Design review of the part built by this model. Coordinates are the model's own, in mm. Round coordinates to 2 decimals unless told otherwise and drop trailing zeros. Loops run counter-clockwise (first coordinate to the right, second up) from the corner with the lowest first, then second, coordinate; pieces in that order, holes last. Notation, with made-up numbers: (79.5, 49.5) - (85.5, 49.5) arc R14 ccw to (85.5, 67.5) - close; hole circle Ø6 at (82.5, -19.5). An arc over 180 degrees is marked (long way). Use one line per item in the form item = value. Start each with the question number.
(1) For pin 1 (4 mm diameter, centred on x = 507.5, z = 30, fed in from -Y); pin 2 (3.5 mm diameter, centred on x = -250, y = 337.5, fed in from +Z), all flat-tipped, find the tip position at first contact; note any pin that passes through.
(2) Wall thickness on probe 1 along X at (y, z) = (337.5, 28.5); probe 2 along Y at (x, z) = (-250, 28); probe 3 along X at (y, z) = (-359.5, 22): over which ranges is each line inside the solid? List them lowest first. Write a range as [from, to].
(3) We need section C-C, the plane x = -824.5. Write out the cut boundary in (y, z), then the cut area to 3 significant figures.
(4) We need section B-B, the plane x = -308. Write out the cut boundary in (y, z), then the cut area to 3 significant figures.
(5) We need section A-A, the plane z = 13. Write out the cut boundary in (x, y).
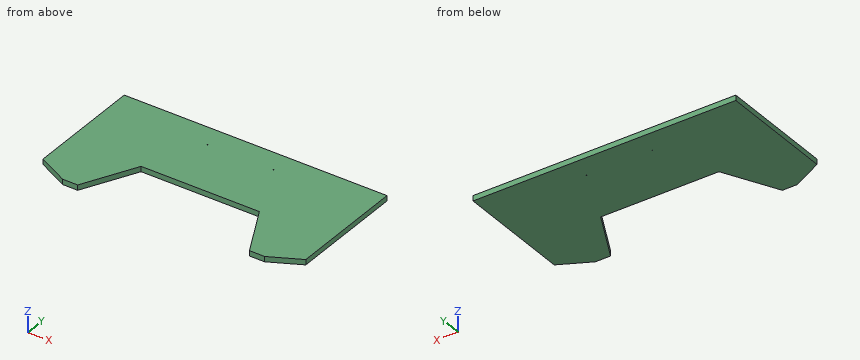
from build123d import *

# Parameters (mm, degrees)
F0_W     = 2000
F0_H     = 1005
F1_DEPTH = 40
F3_DEPTH = 40.001
F5_R     = 3
F6_DEPTH = 40.001
F8_DEPTH = 40.001


with BuildPart() as f1:
    # F0 (on Top) → F1 (new body)
    with BuildSketch(Plane.XY):
        Rectangle(F0_W, F0_H)
    extrude(amount=F1_DEPTH)

    # F2 (on face) → F3 (cut, through all)
    with BuildSketch(Plane.XY.offset(40)):
        Polygon((-450, -102.5), (-653.81018, -502.5), (0, -502.5), (653.81018, -502.5), (450, -102.5), (0, -102.5), align=None)
    extrude(amount=-F3_DEPTH, mode=Mode.SUBTRACT)

    # F5 (on face) → F6 (cut, through all)
    with BuildSketch(Plane(origin=(0, 0, 0), x_dir=(1, 0, 0), z_dir=(0, 0, -1))):
        with Locations((-250, -337.5)):
            Circle(F5_R)
        with Locations((250, -337.5)):
            Circle(F5_R)
    extrude(amount=-F6_DEPTH, mode=Mode.SUBTRACT)

    # F7 (on face) → F8 (cut, through all)
    with BuildSketch(Plane.XY.offset(40)):
        Polygon((-768.41196, -502.5), (-1000, -384.5), (-1000, -502.5), align=None)
        Polygon((1000, -502.5), (1000, -384.5), (768.41196, -502.5), align=None)
    extrude(amount=-F8_DEPTH, mode=Mode.SUBTRACT)


solid = f1.part
Data:
q1.pin_1 = -219.28
q1.pin_2 = through
q2.probe_1 = [-1000, -253], [-247, 247], [253, 1000]
q2.probe_2 = [-102.5, 334.5], [340.5, 502.5]
q2.probe_3 = [-1000, -580.95], [580.95, 1000]
q3.outline = (-473.92, 0) - (502.5, 0) - (502.5, 40) - (-473.92, 40) - close
q3.area = 39,100 mm^2
q4.outline = (-102.5, 0) - (502.5, 0) - (502.5, 40) - (-102.5, 40) - close
q4.area = 24,200 mm^2
q5.outline = (-1000, -384.5) - (-768.41, -502.5) - (-653.81, -502.5) - (-450, -102.5) - (450, -102.5) - (653.81, -502.5) - (768.41, -502.5) - (1000, -384.5) - (1000, 502.5) - (-1000, 502.5) - close; hole circle Ø6 at (-250, 337.5); hole circle Ø6 at (250, 337.5)
